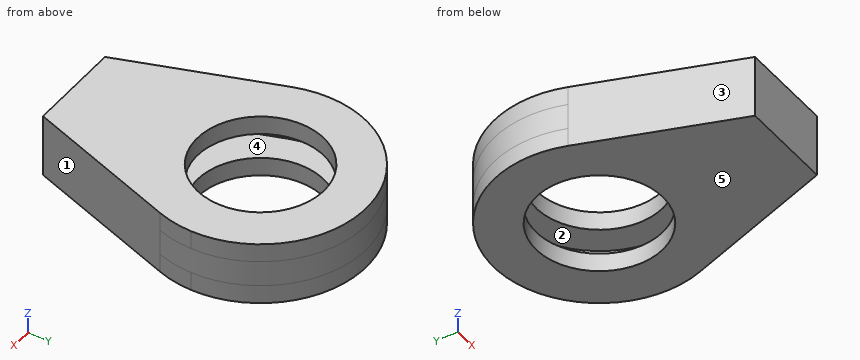
from build123d import *

# Parameters (mm, degrees)
F0_R     = 13.5
F1_DEPTH = 4
F3_DEPTH = 5.5
F4_R     = 13.5
F5_DEPTH = 4


with BuildPart() as f1:
    # F0 (on Top) → F1 (new body)
    with BuildSketch(Plane.XY):
        with BuildLine():
            ThreePointArc((21.255276, -7.379922), (22.186637, -3.742078), (22.5, 0))
            ThreePointArc((22.5, 0), (-3.742078, 22.186637), (-21.255276, -7.379922))
            ThreePointArc((-21.255276, -7.379922), (0, -22.5), (21.255276, -7.379922))
        make_face()
        Circle(F0_R, mode=Mode.SUBTRACT)
        with BuildLine():
            ThreePointArc((21.255276, -7.379922), (0, -22.5), (-21.255276, -7.379922))
            Line((-21.255276, -7.379922), (-10, -39.796796))
            Line((-10, -39.796796), (0, -39.796796))
            Line((0, -39.796796), (10, -39.796796))
            Line((10, -39.796796), (21.255276, -7.379922))
        make_face()
    extrude(amount=F1_DEPTH)

    # F2 (on face) → F3 (join)
    with BuildSketch(Plane.XY.offset(4)):
        with BuildLine():
            Line((10, -39.796796), (21.255276, -7.379922))
            ThreePointArc((21.255276, -7.379922), (0, 22.5), (-21.255276, -7.379922))
            Line((-21.255276, -7.379922), (-10, -39.796796))
            Line((-10, -39.796796), (10, -39.796796))
        make_face()
        with BuildLine():
            ThreePointArc((-18.421239, -6.395932), (-3.243134, 19.228419), (19.5, 0))
            ThreePointArc((19.5, 0), (19.228419, -3.243134), (18.421239, -6.395932))
            Line((18.421239, -6.395932), (10.707315, -28.613186))
            Line((10.707315, -28.613186), (-10.707315, -28.613186))
            Line((-10.707315, -28.613186), (-18.421239, -6.395932))
        make_face(mode=Mode.SUBTRACT)
    extrude(amount=F3_DEPTH)

    # F4 (on face) + F0 (on Top) → F5 (join)
    with BuildSketch(Plane.XY.offset(9.5)):
        with BuildLine():
            ThreePointArc((21.255276, -7.379922), (22.186637, -3.742078), (22.5, 0))
            ThreePointArc((22.5, 0), (-3.742078, 22.186637), (-21.255276, -7.379922))
            ThreePointArc((-21.255276, -7.379922), (0, -22.5), (21.255276, -7.379922))
        make_face()
        Circle(F4_R, mode=Mode.SUBTRACT)
        with BuildLine():
            ThreePointArc((21.255276, -7.379922), (0, -22.5), (-21.255276, -7.379922))
            Line((-21.255276, -7.379922), (-10, -39.796796))
            Line((-10, -39.796796), (0, -39.796796))
            Line((0, -39.796796), (10, -39.796796))
            Line((10, -39.796796), (21.255276, -7.379922))
        make_face()
    with BuildSketch(Plane.XY):
        with BuildLine():
            ThreePointArc((21.255276, -7.379922), (22.186637, -3.742078), (22.5, 0))
            ThreePointArc((22.5, 0), (-3.742078, 22.186637), (-21.255276, -7.379922))
            ThreePointArc((-21.255276, -7.379922), (0, -22.5), (21.255276, -7.379922))
        make_face()
        Circle(F0_R, mode=Mode.SUBTRACT)
        with BuildLine():
            ThreePointArc((21.255276, -7.379922), (0, -22.5), (-21.255276, -7.379922))
            Line((-21.255276, -7.379922), (-10, -39.796796))
            Line((-10, -39.796796), (0, -39.796796))
            Line((0, -39.796796), (10, -39.796796))
            Line((10, -39.796796), (21.255276, -7.379922))
        make_face()
    extrude(amount=F5_DEPTH)


solid = f1.part
Design review of the part built by this model. Coordinates are the model's own, in mm. Face numbers are marked on the shaded views. A direction names the side the tool comes from. Round coordinates to 2 decimals unless told otherwise and drop trailing zeros. Write each loop counter-clockwise with the first axis right and the second up, starting at its lowest first coordinate (ties: lowest second). Pieces come first, ordered by that corner, then holes. Notation, with made-up numbers: (4, -14.5) - (54, -14.5) arc R20 ccw to (54, 15.5) - close; hole circle Ø1 at (49, 36). An arc over 180 degrees is marked (long way). Return JSON: item names as keys, results as strings. Group by question number.
Item 1: We need section C-C on y = -9.5. Write out the cut boundary in (x, z).
Item 2: We need section D-D on x = 17. Write out the cut boundary in (y, z), and give its area (3 significant figures).
Item 3: Machinability: for the marked faces 1 and 2, which of the approach directions +Z, -Z, +X, -X, +Y, -Y give a long, thin tool a straight path to every point of the face, cutting with its end or side? Answer none if there is none.
Item 4: We need section A-A on x = 0. Write out the cut boundary in (y, z).
Item 5: We need section B-B on z = 6. Write out the cut boundary in (x, y).
Item 6: The part is to be moulded in two halves that separate along Z. For the marked faces 3, 4 and 5, say which applies: pulls with the +Z half, pulls with the -Z half, needs draft (parallel to the pull), parting line crosses it, or undercut.
Item 7: Insertion check: P1, Ø24.5, axis at x = 0, y = 0, coming from the -Z side; P2, Ø4, axis at y = 12.5, z = 9.5, coming from the -X side; P3, Ø6, axis at y = -32, z = 4.5, coming from the +X side; P4, Ø2, axis at x = -5.5, z = 12, coming from the +Y side. Each pin has a flat end and moves straight along its axis. Give the tip position at first contact, or say it passes through.
Item 8: For probe 1 along Z at (x, y) = (14, -9.5); probe 2 along Y at (x, z) = (0, 10.8); probe 3 along X at (y, z) = (0, 6.3), list the stretches that pass through material, from the lowest coordinate up. Write a range as [from, to].
Model answer:
{
 "1": {"outline": "(-20.52, 0) - (-9.59, 0) - (-9.59, 4) - (-17.34, 4) - (-17.34, 9.5) - (-9.59, 9.5) - (-9.59, 13.5) - (-20.52, 13.5) - close; (9.59, 0) - (20.52, 0) - (20.52, 13.5) - (9.59, 13.5) - (9.59, 9.5) - (17.34, 9.5) - (17.34, 4) - (9.59, 4) - close"},
 "2": {"outline": "(-19.64, 0) - (14.74, 0) - (14.74, 13.5) - (-19.64, 13.5) - close; hole (-10.49, 4) - (9.55, 4) - (9.55, 9.5) - (-10.49, 9.5) - close", "area": "354 mm²"},
 "3": {"face 1": "+Z, -Z, +X, -Y", "face 2": "none"},
 "4": {"outline": "(-39.8, 0) - (-13.5, 0) - (-13.5, 4) - (-28.61, 4) - (-28.61, 9.5) - (-13.5, 9.5) - (-13.5, 13.5) - (-39.8, 13.5) - close; (13.5, 0) - (22.5, 0) - (22.5, 13.5) - (13.5, 13.5) - (13.5, 9.5) - (19.5, 9.5) - (19.5, 4) - (13.5, 4) - close"},
 "5": {"outline": "(-21.26, -7.38) - (-10, -39.8) - (10, -39.8) - (21.26, -7.38) arc R22.5 ccw (long way) to start; hole (-18.42, -6.4) - (-10.71, -28.61) - (10.71, -28.61) - (18.42, -6.4) arc R19.5 ccw to (19.5, 0) arc R19.5 ccw (long way) to start"},
 "6": {"face 3": "needs draft", "face 4": "undercut", "face 5": "pulls with the -Z half"},
 "7": {"P1": "passes through", "P2": "stops at x = -19.9", "P3": "stops at x = 13.75", "P4": "stops at y = 22.05"},
 "8": {"probe 1": "z = [0, 4], [9.5, 13.5]", "probe 2": "y = [-39.8, -13.5], [13.5, 22.5]", "probe 3": "x = [-22.5, -19.5], [19.5, 22.5]"}
}
